Part model, mm, in its own coordinate system. A direction names the side the tool comes from. Coordinates: 2 decimals unless noted, no trailing zeros. Loops run counter-clockwise (first coordinate to the right, second up) from the corner with the lowest first, then second, coordinate; pieces in that order, holes last. Notation, with made-up numbers: (50, -11.5) - (109, -11.5) arc R16 cw to (109, -0.5) - close; hole circle Ø7 at (50.25, 17). An arc over 180 degrees is marked (long way). Use a Markdown table: item, result. Add a question column.
1. Pull direction Z, two halves, no side cores. Call faces 1 (the flat face through (73.57, -1.57, 18.83)), 2 (the cylindrical face through (89.313, -1.565, -57.505)), 3 (the flat face through (0, -3.175, -113)): pulls with the +Z half, pulls with the -Z half, needs draft (parallel to the pull), parting line crosses it, or undercut.
2. Wall check: probe 1 along Z at (x, y) = (13, -2.55); probe 2 along Z at (x, y) = (7, -2.4); probe 3 along Z at (x, y) = (-125, -0.4). Give the ranges that are in metal, low to high. Write a range as [from, to].
3. 3-axis set-ups, long thin cutter, end or side, ignore diameter. For faces 4 (the cylindrical face through (89.694, -1.565, -174.346)), 5 (the flat face through (0, 0, -113)), 6 (the flat face through (-0.239, -1.565, -224.096)): which of +Z, -Z, +X, -X, +Y, -Y reach the whole face in a straight line?
4. Drop flat-ended pins along their axis: pin 1 (1.5 mm diameter, centred on y = -2.5, z = -120, fed in from +X); pin 2 (1 mm diameter, centred on y = -1.5, z = -116, fed in from -X); pin 3 (1 mm diameter, centred on x = -97.5, y = -2, fed in from -Z). Give the stop position or say it passes through.
5. Band-saw the part on D-D, the plane y = -2. Count the separate pieces of the cut face and the enclosed holes in it, plus the area to 3 significant figures.
6. Band-saw the part on A-A, the plane x = -93. Give the cut face in (y, z) (3 decimals), plus the area to 3 significant figures.
7. Band-saw the part on C-C, the plane x = 15.5. Give the cut face in (y, z) (3 decimals), plus the area to 3 significant figures.
8. Band-saw the part on B-B, the plane z = -278. Give the cut face in (x, y) (3 decimals), plus the area to 3 significant figures.
from build123d import *

# Parameters (mm, degrees)
F0_R     = 16.51
F1_DEPTH = 3.175


# Not quite as in the source:
# - ends of sketch curves that miss each other by under 0.0002 mm in the source are joined
# - a feature names something its author has since deleted; it is built from what else it names


with BuildPart() as f1:
    # F0 (on Front) → F1 (new body)
    with BuildSketch(Plane.XZ):
        with BuildLine():
            Line((72.172606051, -154.628444229), (72.172606051, -76.840944229))
            Line((72.172606051, -76.840944229), (72.172606051, -64.494198626))
            ThreePointArc((72.172606051, -64.494198626), (89.5045003647, -57.3150929397), (96.683606051, -39.983198626))
            Line((96.683606051, -39.983198626), (96.683606051, -30.0584486086))
            Line((96.683606051, -30.0584486086), (49.8026024117, 69.0988139849))
            Line((49.8026024117, 69.0988139849), (44.4719158113, 81.3992435336))
            Line((44.4719158113, 81.3992435336), (-29.9480052508, 81.3992435336))
            Line((-29.9480052508, 81.3992435336), (-35.9978974571, 50.6829957967))
            Line((-35.9978974571, 50.6829957967), (-19.4879078689, 50.6714224456))
            ThreePointArc((-19.4879078689, 50.6714224456), (-15.5812211009, 47.1637298884), (-13.9720730804, 42.1660573792))
            Line((-13.9720730804, 42.1660573792), (-5.4024819992, 38.3506346508))
            Line((-5.4024819992, 38.3506346508), (-2.9009456417, 36.1038269705))
            Line((-2.9009456417, 36.1038269705), (-2.3647786124, 27.9011076368))
            ThreePointArc((-2.3647786124, 27.9011076368), (3.4353485173, 23.5426794776), (4.3712937617, 16.3481414632))
            Line((4.3712937617, 16.3481414632), (4.2880811809, 16.2515226396))
            Line((4.2880811809, 16.2515226396), (4.2880776677, 1.0115236557))
            Line((4.2880776677, 1.0115236557), (-4.6405893252, -15.5276898319))
            Line((-4.6405893252, -15.5276898319), (-123.1544493252, -15.5276898319))
            ThreePointArc((-123.1544493252, -15.5276898319), (-147.6377037222, -40.010944229), (-123.1544493252, -64.494198626))
            Line((-123.1544493252, -64.494198626), (-81.4537847014, -64.494198626))
            Line((-81.4537847014, -64.494198626), (-81.4537847014, -76.840944229))
            Line((-81.4537847014, -76.840944229), (-81.4537847014, -154.628444229))
            Line((-81.4537847014, -154.628444229), (-81.4537847014, -166.9751898319))
            Line((-81.4537847014, -166.9751898319), (-123.1544493252, -166.9751898319))
            ThreePointArc((-123.1544493252, -166.9751898319), (-147.6377037222, -191.458444229), (-123.1544493252, -215.941698626))
            Line((-123.1544493252, -215.941698626), (-4.6405893252, -215.941698626))
            Line((-4.6405893252, -215.941698626), (4.2880776677, -232.4809121137))
            Line((4.2880776677, -232.4809121137), (4.2880811809, -247.7209110976))
            Line((4.2880811809, -247.7209110976), (4.3712937617, -247.8175299212))
            ThreePointArc((4.3712937617, -247.8175299212), (3.4353485173, -255.0120679356), (-2.3647786124, -259.3704960948))
            Line((-2.3647786124, -259.3704960948), (-2.9009456417, -267.5732154285))
            Line((-2.9009456417, -267.5732154285), (-5.4024819992, -269.8200231088))
            Line((-5.4024819992, -269.8200231088), (-13.9720735102, -273.6354510709))
            ThreePointArc((-13.9720735102, -273.6354510709), (-15.5812211009, -278.6331183464), (-19.487905219, -282.1408109018))
            Line((-19.487905219, -282.1408109018), (-35.9978974571, -282.1523842547))
            Line((-35.9978974571, -282.1523842547), (-29.9480052508, -312.8686319916))
            Line((-29.9480052508, -312.8686319916), (44.4719158113, -312.8686319916))
            Line((44.4719158113, -312.8686319916), (49.8026024117, -300.5682024429))
            Line((49.8026024117, -300.5682024429), (96.683606051, -201.4109398494))
            Line((96.683606051, -201.4109398494), (96.683606051, -191.4861898319))
            ThreePointArc((96.683606051, -191.4861898319), (89.5045003647, -174.1542955183), (72.172606051, -166.9751898319))
            Line((72.172606051, -166.9751898319), (72.172606051, -154.628444229))
        make_face()
        with Locations((11.6086210255, -285.7798588113)):
            Circle(F0_R, mode=Mode.SUBTRACT)
        with Locations((11.6086210255, 54.3104703533)):
            Circle(F0_R, mode=Mode.SUBTRACT)
    extrude(amount=F1_DEPTH)


solid = f1.part
Geometry check:
| question | item | result |
|---|---|---|
| 1 | face 1 | pulls with the +Z half |
| 1 | face 2 | undercut |
| 1 | face 3 | needs draft |
| 2 | probe 1 | z = [-312.87, -302.23], [-269.33, 37.86], [70.76, 81.4] |
| 2 | probe 2 | z = [-312.87, -301.63], [-269.93, 38.46], [70.16, 81.4] |
| 2 | probe 3 | z = [-215.87, -167.04], [-64.42, -15.6] |
| 3 | face 4 | +X, +Y, -Y |
| 3 | face 5 | +Z, -Z, +X, -X, +Y |
| 3 | face 6 | -X, +Y, -Y |
| 4 | pin 1 | stops at x = 72.17 |
| 4 | pin 2 | stops at x = -81.45 |
| 4 | pin 3 | stops at z = -215.94 |
| 5 | separate pieces | 1 |
| 5 | enclosed holes | 2 |
| 5 | area | 52,300 mm^2 |
| 6 | outline | (-3.175, -215.942) - (0, -215.942) - (0, -166.975) - (-3.175, -166.975) - close; (-3.175, -64.494) - (0, -64.494) - (0, -15.528) - (-3.175, -15.528) - close |
| 6 | area | 311 mm^2 |
| 7 | outline | (-3.175, -312.869) - (0, -312.869) - (0, -301.825) - (-3.175, -301.825) - close; (-3.175, -269.735) - (0, -269.735) - (0, 38.266) - (-3.175, 38.266) - close; (-3.175, 70.355) - (0, 70.355) - (0, 81.399) - (-3.175, 81.399) - close |
| 7 | area | 1,050 mm^2 |
| 8 | outline | (-15.203, -3.175) - (-2.953, -3.175) - (-2.953, 0) - (-15.203, 0) - close; (26.171, -3.175) - (60.473, -3.175) - (60.473, 0) - (26.171, 0) - close |
| 8 | area | 148 mm^2 |
